Geometry: final body of the model. Coordinates: model frame, mm. A direction names the side the tool comes from. Coordinates: 2 decimals unless noted, no trailing zeros. Write each loop counter-clockwise with the first axis right and the second up, starting at its lowest first coordinate (ties: lowest second). Pieces come first, ordered by that corner, then holes. Notation, with made-up numbers: (47.25, 35) - (56.25, 35) arc R29 ccw to (56.25, 73) - close; hole circle Ø2 at (10.25, 8.5). An arc over 180 degrees is marked (long way). Answer as a JSON object with one key per item and string values. Group by question number.
Item 1: Section B-B on y = 89. Return loops of the section in (x, z).
Item 2: Mould query, pull axis Y, two halves, no side actions, for faces 1 (the flat face through (86, 5.75, 4)), 2 (the flat face through (109.75, 88, 4)), 3 (the flat face through (29, 52.25, 4)), 4 (the flat face through (85, 45, 2)). Classes: pulls with the +Y half, pulls with the -Y half, needs draft (parallel to the pull), parting line crosses it, or undercut.
Item 3: Line query: line 1 along X through (y, z) = (85, 2.7); line 2 along Y through (x, z) = (152, 2.05); line 3 along Z through (x, y) = (98, 46.5). Output: solid intervals per line, ascending. Write a range as from..to.
Item 4: Section A-A on z = 4.35. Return loops of the section in (x, y).
Item 5: First-contact query: pin 1 Ø3.5 at (x, y) = (2, 28) entering from -Z; pin 2 Ø0.9 at (x, z) = (112, 4.5) entering from +Y; pin 3 Ø0.9 at (y, z) = (4.5, 5) entering from +X. Flat tips, straight axial feed; report the tip coordinate or a pass-through.
Item 6: Section D-D on y = 24. Return loops of the section in (x, z).
Item 7: Set-up query: faces 5 (the flat face through (63.25, 88, 4)), 6 (the flat face through (29, 5.75, 4)), 7 (the flat face through (29, 55.25, 4)), 8 (the flat face through (112.75, 88, 4)), 9 (the flat face through (29, 2.75, 4)). Return all of +Z, -Z, +X, -X, +Y, -Y with unobstructed straight access to the full face (end or side cutting, diameter ignored); none if empty.
Item 8: Section C-C on x = 138. Return loops of the section in (y, z), and give its area (3 significant figures).
```python
from build123d import *

# Parameters (mm, degrees)
BOX010_W     = 3
BOX010_H     = 58
BOX010_DEPTH = 1
BOX009_W     = 3
BOX009_H     = 58
BOX009_DEPTH = 1
BOX008_W     = 20
BOX008_H     = 3
BOX008_DEPTH = 6
BOX007_W     = 20
BOX007_H     = 3
BOX007_DEPTH = 6
BOX006_W     = 20
BOX006_H     = 3
BOX006_DEPTH = 6
BOX005_W     = 20
BOX005_H     = 3
BOX005_DEPTH = 6
BOX004_W     = 20
BOX004_H     = 3
BOX004_DEPTH = 6
BOX003_W     = 20
BOX003_H     = 3
BOX003_DEPTH = 6
BOX002_W     = 20
BOX002_H     = 3
BOX002_DEPTH = 6
BOX001_W     = 110
BOX001_H     = 58
BOX001_DEPTH = 2
BOX_W        = 165
BOX_H        = 58
BOX_DEPTH    = 2
BOX011_W     = 3
BOX011_H     = 58
BOX011_DEPTH = 1


with BuildPart() as cube010:
    # Box010 → Box010 (new body)
    with BuildSketch(Plane(origin=(169, 0, 1), x_dir=(1, 0, 0), z_dir=(0, 0, 1))):
        with Locations((1.5, 29)):
            Rectangle(BOX010_W, BOX010_H)
    extrude(amount=BOX010_DEPTH)


with BuildPart() as cube009:
    # Box009 → Box009 (new body)
    with BuildSketch(Plane(origin=(1, 0, 1), x_dir=(1, 0, 0), z_dir=(0, 0, 1))):
        with Locations((1.5, 29)):
            Rectangle(BOX009_W, BOX009_H)
    extrude(amount=BOX009_DEPTH)


with BuildPart() as cube008:
    # Box008 → Box008 (new body)
    with BuildSketch(Plane(origin=(112.75, 78.5, 0), x_dir=(0, 1, 0), z_dir=(0, 0, 1))):
        with Locations((10, 1.5)):
            Rectangle(BOX008_W, BOX008_H)
    extrude(amount=BOX008_DEPTH)


with BuildPart() as cube007:
    # Box007 → Box007 (new body)
    with BuildSketch(Plane(origin=(63.25, 78.5, 0), x_dir=(0, 1, 0), z_dir=(0, 0, 1))):
        with Locations((10, 1.5)):
            Rectangle(BOX007_W, BOX007_H)
    extrude(amount=BOX007_DEPTH)


with BuildPart() as cube006:
    # Box006 → Box006 (new body)
    with BuildSketch(Plane(origin=(134.83, 52.25, 0), x_dir=(1, 0, 0), z_dir=(0, 0, 1))):
        with Locations((10, 1.5)):
            Rectangle(BOX006_W, BOX006_H)
    extrude(amount=BOX006_DEPTH)


with BuildPart() as cube005:
    # Box005 → Box005 (new body)
    with BuildSketch(Plane(origin=(18.67, 52.25, 0), x_dir=(1, 0, 0), z_dir=(0, 0, 1))):
        with Locations((10, 1.5)):
            Rectangle(BOX005_W, BOX005_H)
    extrude(amount=BOX005_DEPTH)


with BuildPart() as cube004:
    # Box004 → Box004 (new body)
    with BuildSketch(Plane(origin=(134.83, 2.75, 0), x_dir=(1, 0, 0), z_dir=(0, 0, 1))):
        with Locations((10, 1.5)):
            Rectangle(BOX004_W, BOX004_H)
    extrude(amount=BOX004_DEPTH)


with BuildPart() as cube003:
    # Box003 → Box003 (new body)
    with BuildSketch(Plane(origin=(76.34, 2.75, 0), x_dir=(1, 0, 0), z_dir=(0, 0, 1))):
        with Locations((10, 1.5)):
            Rectangle(BOX003_W, BOX003_H)
    extrude(amount=BOX003_DEPTH)


with BuildPart() as cube002:
    # Box002 → Box002 (new body)
    with BuildSketch(Plane(origin=(18.67, 2.75, 0), x_dir=(1, 0, 0), z_dir=(0, 0, 1))):
        with Locations((10, 1.5)):
            Rectangle(BOX002_W, BOX002_H)
    extrude(amount=BOX002_DEPTH)


with BuildPart() as cube001:
    # Box001 → Box001 (new body)
    with BuildSketch(Plane(origin=(115.5, 0, 0), x_dir=(0, 1, 0), z_dir=(0, 0, 1))):
        with Locations((55, 29)):
            Rectangle(BOX001_W, BOX001_H)
    extrude(amount=BOX001_DEPTH)


with BuildPart() as cube:
    # Box → Box (new body)
    with BuildSketch(Plane(origin=(4, 0, 0), x_dir=(1, 0, 0), z_dir=(0, 0, 1))):
        with Locations((82.5, 29)):
            Rectangle(BOX_W, BOX_H)
    extrude(amount=BOX_DEPTH)


with BuildPart() as fusion:
    # Box011 → Box011 (new body)
    with BuildSketch(Plane(origin=(115.5, 110, 1), x_dir=(0, 1, 0), z_dir=(0, 0, 1))):
        with Locations((1.5, 29)):
            Rectangle(BOX011_W, BOX011_H)
    extrude(amount=BOX011_DEPTH)

    # Fusion: union Cube010, Cube009, Cube008, Cube007, Cube006, Cube005, Cube004, Cube003, Cube002, Cube001, Cube
    add(cube010.part)
    add(cube009.part)
    add(cube008.part)
    add(cube007.part)
    add(cube006.part)
    add(cube005.part)
    add(cube004.part)
    add(cube003.part)
    add(cube002.part)
    add(cube001.part)
    add(cube.part)


solid = fusion.part
```
Checks:
{
 "1": {"outline": "(57.5, 0) - (115.5, 0) - (115.5, 2) - (112.75, 2) - (112.75, 6) - (109.75, 6) - (109.75, 2) - (63.25, 2) - (63.25, 6) - (60.25, 6) - (60.25, 2) - (57.5, 2) - close"},
 "2": {"face 1": "pulls with the +Y half", "face 2": "needs draft", "face 3": "undercut", "face 4": "undercut"},
 "3": {"line 1": "60.25..63.25, 109.75..112.75", "line 2": "2.75..5.75, 52.25..55.25", "line 3": "0..2"},
 "4": {"outline": "(18.67, 2.75) - (38.67, 2.75) - (38.67, 5.75) - (18.67, 5.75) - close; (18.67, 52.25) - (38.67, 52.25) - (38.67, 55.25) - (18.67, 55.25) - close; (60.25, 78.5) - (63.25, 78.5) - (63.25, 98.5) - (60.25, 98.5) - close; (76.34, 2.75) - (96.34, 2.75) - (96.34, 5.75) - (76.34, 5.75) - close; (109.75, 78.5) - (112.75, 78.5) - (112.75, 98.5) - (109.75, 98.5) - close; (134.83, 2.75) - (154.83, 2.75) - (154.83, 5.75) - (134.83, 5.75) - close; (134.83, 52.25) - (154.83, 52.25) - (154.83, 55.25) - (134.83, 55.25) - close"},
 "5": {"pin 1": "z = 1", "pin 2": "y = 98.5", "pin 3": "x = 154.83"},
 "6": {"outline": "(1, 1) - (4, 1) - (4, 0) - (169, 0) - (169, 1) - (172, 1) - (172, 2) - (1, 2) - close"},
 "7": {"face 5": "+Z, +Y, -Y", "face 6": "+Z, +X, -X", "face 7": "+Z, +X, -X, +Y", "face 8": "+Z, +X, +Y, -Y", "face 9": "+Z, +X, -X, -Y"},
 "8": {"outline": "(0, 0) - (58, 0) - (58, 2) - (55.25, 2) - (55.25, 6) - (52.25, 6) - (52.25, 2) - (5.75, 2) - (5.75, 6) - (2.75, 6) - (2.75, 2) - (0, 2) - close", "area": "140 mm^2"}
}
